```python
from build123d import *

# Parameters (mm, degrees)
SKETCH1_R           = 2.5
BOSS_EXTRUDE1_DEPTH = 26.5
SKETCH2_R           = 4
BOSS_EXTRUDE2_DEPTH = 4.5
CHAMFER1_SIZE       = 0.3


with BuildPart() as part:
    # Sketch1 → Boss-Extrude1 (new body)
    with BuildSketch(Plane.XY):
        Circle(SKETCH1_R)
    extrude(amount=BOSS_EXTRUDE1_DEPTH)

    # Sketch2 → Boss-Extrude2 (add)
    with BuildSketch(Plane.XY.offset(26.5)):
        Circle(SKETCH2_R)
    extrude(amount=BOSS_EXTRUDE2_DEPTH)

    # Chamfer1
    chamfer1_edges = [part.edges().sort_by_distance(p)[0] for p in [
        (-2.5, 0, 0),
        (-4, 0, 26.5),
        (-4, 0, 31),
    ]]
    chamfer(chamfer1_edges, length=CHAMFER1_SIZE)


solid = part.part
```
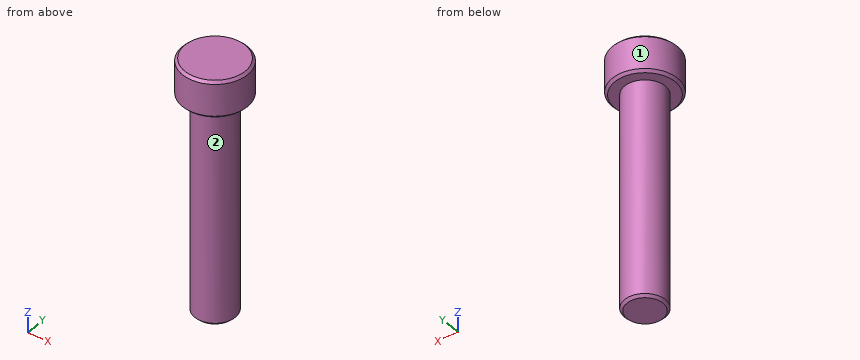
For this review, take the finished solid that the model builds, in its own axes (mm). Face numbers are marked on the shaded views. A direction names the side the tool comes from. Coordinates: 2 decimals unless noted, no trailing zeros. Loops run counter-clockwise (first coordinate to the right, second up) from the corner with the lowest first, then second, coordinate; pieces in that order, holes last.
1. Insertion check: P1, Ø1, axis at x = 1.5, z = 19, coming from the -Y side; P2, Ø2, axis at y = -1, z = 13, coming from the +X side; P3, Ø2, axis at y = -1, z = 16, coming from the -X side. Each pin has a flat end and moves straight along its axis. Give the tip position at first contact, or say it passes through.
2. Add section A-A, the plane x = 0. Give the boundary of the cut face in (y, z), then the cut area to 3 significant figures.
3. For the marked faces 1 and 2, list the 3-axis set-ups (+Z, -Z, +X, -X, +Y, -Y) from which the entire face can be reached by the end or side of a thin tool; tool diameter is ignored.
4. Add section C-C, the plane z = 23. Give the boundary of the cut face in (x, y).
5. For line 1 (Z direction, x = 0, y = 3); line 2 (Y direction, x = 1, z = 7); line 3 (Z direction, x = 1.75, y = 1.75), list the stretches that pass through material, from the lowest coordinate up.
Result:
1. P1: stops at y = -2.29
1. P2: stops at x = 2.5
1. P3: stops at x = -2.5
2. outline: (-4, 26.8) - (-3.7, 26.5) - (-2.5, 26.5) - (-2.5, 0.3) - (-2.2, 0) - (2.2, 0) - (2.5, 0.3) - (2.5, 26.5) - (3.7, 26.5) - (4, 26.8) - (4, 30.7) - (3.7, 31) - (-3.7, 31) - (-4, 30.7) - close
2. area: 168 mm2
3. face 1: +Z, -Z
3. face 2: -Z
4. outline: circle Ø5 at (0, 0)
5. line 1: z = 26.5 to 31
5. line 2: y = -2.29 to 2.29
5. line 3: z = 0.27 to 31
